Here's how the part is built. I have some questions about the finished solid (model axes, mm). Round coordinates to 2 decimals unless told otherwise and drop trailing zeros. Loops run counter-clockwise (first coordinate to the right, second up) from the corner with the lowest first, then second, coordinate; pieces in that order, holes last. Notation, with made-up numbers: (52, 12) - (109, 12) arc R17 cw to (109, 28) - close; hole circle Ø7 at (-9, 3.5). An arc over 180 degrees is marked (long way). Answer as a JSON object with one key per item and string values. Group by question number.
1) I want a section at D-D, the plane z = 27. Please give me the cut outline in (x, y).
2) Will these pins go through, and if not, where does the flat tip stop? P1, Ø1, axis at x = 57, z = -21.5, coming from the -Y side; P2, Ø1.5, axis at x = 84.5, y = 2.5, coming from the -Z side; P3, Ø2.5, axis at y = 2, z = 2.5, coming from the +X side; P4, Ø3.5, axis at y = 3.5, z = -43, coming from the +X side.
3) I want a section at A-A, the plane z = 2. Please give me the cut outline in (x, y).
4) If I drill on line 1 along Z through (x, y) = (80, 2.5); line 2 along Z through (x, y) = (83.5, 1.5); line 3 along Z through (x, y) = (56.5, 1.5), over which ranges is the centre line in solid material (lowest first)? Write a range as [from, to].
5) I want a section at B-B, the plane x = 32. Please give me the cut outline in (y, z), then the cut area to 3 significant figures.
6) I want a section at C-C, the plane y = 6.5. Please give me the cut outline in (x, z).
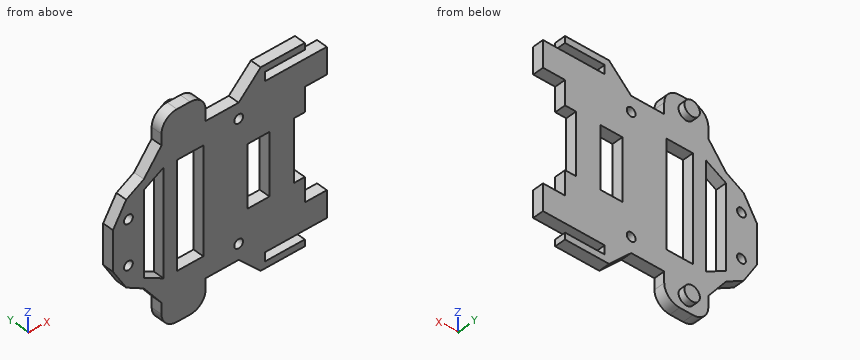
from build123d import *

# Parameters (mm, degrees)
EXTRUDE_1_DEPTH     = 5
SKETCH_2_R          = 2
SKETCH_2_W          = 12
SKETCH_2_H          = 48
SKETCH_2_W_2        = 10
SKETCH_2_H_2        = 28
CUT_EXTRUDE_1_DEPTH = 44
SKETCH_3_R          = 3.5
EXTRUDE_2_DEPTH     = 3
FILLET_1_R          = 7


with BuildPart() as part:
    # 草图1 → 凸台-拉伸1 (new body)
    with BuildSketch(Plane(origin=(0, 0, 0), x_dir=(1, 0, 0), z_dir=(0, 1, 0))):
        Polygon((0, -9), (0, 9), (6, 19), (14, 23.618802154), (22, 34), (22, 46), (42, 46), (42, 34), (57, 34), (67, 44), (87, 44), (87, 41), (69, 41), (69, 37), (97, 37), (97, 25), (87, 25), (87, 14), (82, 14), (82, -14), (87, -14), (87, -25), (97, -25), (97, -37), (69, -37), (69, -41), (87, -41), (87, -44), (67, -44), (57, -34), (42, -34), (42, -46), (22, -46), (22, -34), (14, -23.618802154), (6, -19), align=None)
    extrude(amount=EXTRUDE_1_DEPTH)

    # 草图2 → 切除-拉伸1 (cut)
    with BuildSketch(Plane(origin=(0, 5, 0), x_dir=(1, 0, 0), z_dir=(0, 1, 0))):
        with Locations(Location((7, 10, 0), (0, 0, 270))):
            Circle(SKETCH_2_R)
        with Locations(Location((7, -10, 0), (0, 0, 90))):
            Circle(SKETCH_2_R)
        with Locations(Location((57, 27, 0), (0, 0, 270))):
            Circle(SKETCH_2_R)
        with Locations(Location((57, -27, 0), (0, 0, 90))):
            Circle(SKETCH_2_R)
        Polygon((14, -19), (14, 19), (23, 24), (23, -24), align=None)
        with Locations((35, 0)):
            Rectangle(SKETCH_2_W, SKETCH_2_H)
        with Locations((66, 0)):
            Rectangle(SKETCH_2_W_2, SKETCH_2_H_2)
    extrude(amount=-CUT_EXTRUDE_1_DEPTH, mode=Mode.SUBTRACT)

    # 草图3 → 凸台-拉伸2 (add)
    with BuildSketch(Plane(origin=(0, 5, 0), x_dir=(1, 0, 0), z_dir=(0, 1, 0))):
        with Locations(Location((32, 40, 0), (0, 0, 90))):
            Circle(SKETCH_3_R)
        with Locations(Location((32, -40, 0), (0, 0, 90))):
            Circle(SKETCH_3_R)
    extrude(amount=EXTRUDE_2_DEPTH)

    # 圆角1
    fillet_1_edges = [part.edges().sort_by_distance(p)[0] for p in [
        (22, 2.5, 46),
        (42, 2.5, 46),
        (42, 2.5, -46),
        (22, 2.5, -46),
    ]]
    fillet(fillet_1_edges, radius=FILLET_1_R)


solid = part.part
Outcome:
{
 "1": {"outline": "(16.61, 0) - (55, 0) - (55, 5) - (16.61, 5) - close; (59, 0) - (97, 0) - (97, 5) - (59, 5) - close"},
 "2": {"P1": "y = 0", "P2": "z = -44", "P3": "x = 82", "P4": "x = 87"},
 "3": {"outline": "(0, 0) - (14, 0) - (14, 5) - (0, 5) - close; (23, 0) - (29, 0) - (29, 5) - (23, 5) - close; (41, 0) - (61, 0) - (61, 5) - (41, 5) - close; (71, 0) - (82, 0) - (82, 5) - (71, 5) - close"},
 "4": {"line 1": "[-44, -41], [-37, 37], [41, 44]", "line 2": "[-44, -41], [-37, -14], [14, 37], [41, 44]", "line 3": "[-34, -28.94], [-25.06, 25.06], [28.94, 34]"},
 "5": {"outline": "(0, -46) - (5, -46) - (5, -43.5) - (8, -43.5) - (8, -36.5) - (5, -36.5) - (5, -24) - (0, -24) - close; (0, 24) - (5, 24) - (5, 36.5) - (8, 36.5) - (8, 43.5) - (5, 43.5) - (5, 46) - (0, 46) - close", "area": "262 mm^2"},
 "6": {"outline": "circle Ø7 at (32, -40); circle Ø7 at (32, 40)"}
}
